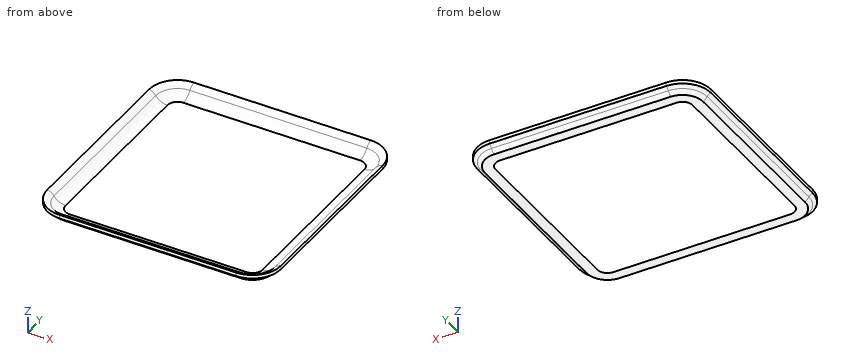
from build123d import *

# Parameters (mm, degrees)
F1_DEPTH = 25
F4_COUNT = 4
F6_ANGLE = 90
F8_COUNT = 4


with BuildPart() as f1:
    # F0 (on Front) → F1 (new body, symmetric)
    with BuildSketch(Plane.XZ):
        with BuildLine():
            ThreePointArc((-27.838012214, 2), (-29.6896524135, 2.4543789583), (-31.1206194405, 3.7142857143))
            ThreePointArc((-31.1206194405, 3.7142857143), (-31.9410332681, 4.5110438468), (-33, 4.9428908461))
            Line((-33, 4.9428908461), (-33, 3.9132711601))
            ThreePointArc((-33, 3.9132711601), (-32.40580245, 3.6171600706), (-31.9412712472, 3.1428571429))
            ThreePointArc((-31.9412712472, 3.1428571429), (-31.4353171545, 2.5273357254), (-30.838012214, 2))
            Line((-30.838012214, 2), (-27.838012214, 2))
        make_face()
    extrude(amount=F1_DEPTH, both=True)


with BuildPart() as f2_1:
    # F2: instance of F1
    add(f1.part.mirror(Plane.YZ))


with BuildPart() as f1_1:
    add(f1.part)

    add(f2_1.part)  # F4 merges F2_1
    # F4: F1, F2_1 ×4 about axis
    f4_axis = Axis((0, 0, 8.481499739), (0, 0, 1))
    for i in range(1, F4_COUNT):
        add(f1.part.rotate(f4_axis, i * 360 / F4_COUNT))
        add(f2_1.part.rotate(f4_axis, i * 360 / F4_COUNT))

    # F4_face (on face) → F6 (revolve)
    with BuildSketch(Plane(origin=(25, -31.316775031, 3.2677689392), x_dir=(0, 1, 0), z_dir=(1, 0, 0))):
        with BuildLine():
            Line((0.478762817, -1.2677689392), (3.478762817, -1.2677689392))
            ThreePointArc((3.478762817, -1.2677689392), (1.6271226175, -0.8133899809), (0.1961555904, 0.4465167751))
            ThreePointArc((0.1961555904, 0.4465167751), (-0.6242582371, 1.2432749076), (-1.683224969, 1.6751219069))
            Line((-1.683224969, 1.6751219069), (-1.683224969, 0.6455022209))
            ThreePointArc((-1.683224969, 0.6455022209), (-1.0890274191, 0.3493911314), (-0.6244962162, -0.1249117963))
            ThreePointArc((-0.6244962162, -0.1249117963), (-0.1185421236, -0.7404332138), (0.478762817, -1.2677689392))
        make_face()
    revolve(axis=Axis((25, -25, -0.1814401951), (0, 0, 1)), revolution_arc=F6_ANGLE)

    # F8: F1 ×4 about axis
    f8_axis = Axis((0, 0, 7.3843663558), (0, 0, 1))


with BuildPart() as f1_2:
    add(f1_1.part)
    for i in range(1, F8_COUNT):
        add(f1_1.part.rotate(f8_axis, i * 360 / F8_COUNT))


solid = f1_2.part
Verification items for the finished model (mm, model axes). Give positions to 0.01 mm unless a question says otherwise; leave off trailing zeros. Order: outer loops, then holes, each group sorted by start corner. A loop starts at its lowest first (then second) coordinate and runs counter-clockwise, first axis right, second up. Notation, with made-up numbers: (60.25, 20) -> (66.25, 20) arc R32 cw to (66.25, 46) -> close; hole circle Ø9 at (20, 45). An arc over 180 degrees is marked (long way). Answer as CSV lines item,"result".
Q1. Sectioned sample at A-A on x = 15. Record the cut outline in (y, z), plus the area to 3 significant figures.
Solutions:
outline,"(-33, 3.91) arc R2 cw to (-31.94, 3.14) arc R5 ccw to (-30.84, 2) -> (-27.84, 2) arc R4 cw to (-31.12, 3.71) arc R3 ccw to (-33, 4.94) -> close; (27.84, 2) -> (30.84, 2) arc R5 ccw to (31.94, 3.14) arc R2 cw to (33, 3.91) -> (33, 4.94) arc R3 ccw to (31.12, 3.71) arc R4 cw to start"
area,"8.21 mm²"
Q2. Scan lines: probe 1 along X at (y, z) = (15, 2.7); probe 2 along Y at (x, z) = (-26, 2.9); probe 3 along Y at (x, z) = (13.5, 4.75). Record each from-to range of solid material in increasing order.
Solutions:
probe 1,"x = -31.59 to -30.1, 30.1 to 31.59"
probe 2,"y = -31.69 to -30.27, 30.27 to 31.69"
probe 3,"y = -33 to -32.38, 32.38 to 33"
